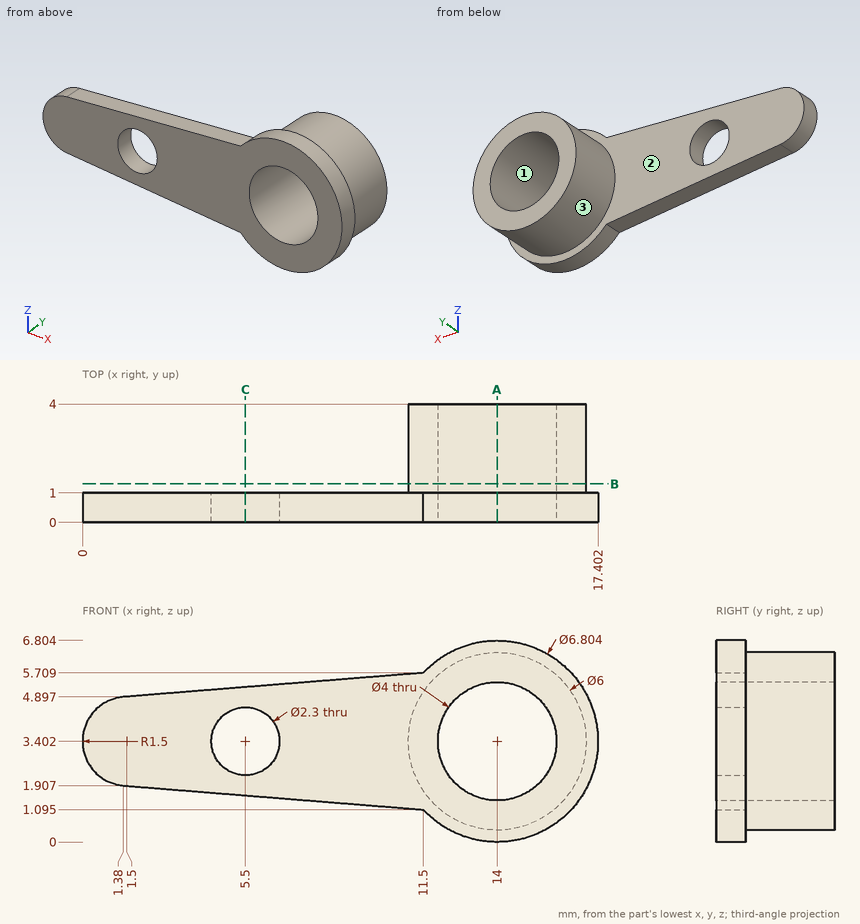
Study the drawing (mm; zero at the part's minimum x, y, z) and answer. Coordinates: 2 decimals unless noted, no trailing zeros. Write each loop counter-clockwise with the first axis right and the second up, starting at its lowest first coordinate (ties: lowest second). Pieces come first, ordered by that corner, then holes.
Q1. Find the intervals of material crossed by line 1 along Z through (x, y) = (14, 1.9); line 2 along Y through (x, z) = (8.5, 1.5); line 3 along X through (y, z) = (0.35, 3.25) (1 decimal), in increasing order.
Returned:
line 1: z = 0.4 to 1.4, 5.4 to 6.4
line 2: y = 0 to 1
line 3: x = 0 to 4.4, 6.6 to 12, 16 to 17.4
Q2. Section A-A, the plane x = 14 is taken. Write down the section's boundary in (y, z) (1 decimal).
Returned:
outline: (0, 0) - (1, 0) - (1, 0.4) - (4, 0.4) - (4, 1.4) - (0, 1.4) - close; (0, 5.4) - (4, 5.4) - (4, 6.4) - (1, 6.4) - (1, 6.8) - (0, 6.8) - close
Q3. The mould has two halves that part along X. Classify the marked faces 1, 2 and 3: released by +X, released by -X, zero draft, split by the parting line, or undercut.
Returned:
face 1: undercut
face 2: zero draft
face 3: split by the parting line
Q4. Section B-B, the plane y = 1.3 is taken. Write down the section's boundary in (x, z), then the cut area to 3 significant figures.
Returned:
outline: circle Ø6 at (14, 3.4); hole circle Ø4 at (14, 3.4)
area: 15.7 mm2
Q5. Given P1, Ø4, axis at x = 2.5, z = 1, coming from the -Y side; P2, Ø1, axis at x = 3, z = 1, coming from the -Y side; P3, Ø1.5, axis at x = 7.5, z = 1.5, coming from the +Y side, each flat-ended and moving along its own axis, determine where each tip first touches the part or whether it passes through.
Returned:
P1: stops at y = 0
P2: passes through
P3: stops at y = 1
Q6. Section C-C, the plane x = 5.5 is taken. Write down the section's boundary in (y, z).
Returned:
outline: (0, 1.58) - (1, 1.58) - (1, 2.25) - (0, 2.25) - close; (0, 4.55) - (1, 4.55) - (1, 5.23) - (0, 5.23) - close
